Check sheet for the drawn part. Datum: minimum x, y, z corner. Units: mm. Round coordinates to 2 decimals unless told otherwise and drop trailing zeros. Order: outer loops, then holes, each group sorted by start corner. A loop starts at its lowest first (then second) coordinate and runs counter-clockwise, first axis right, second up.
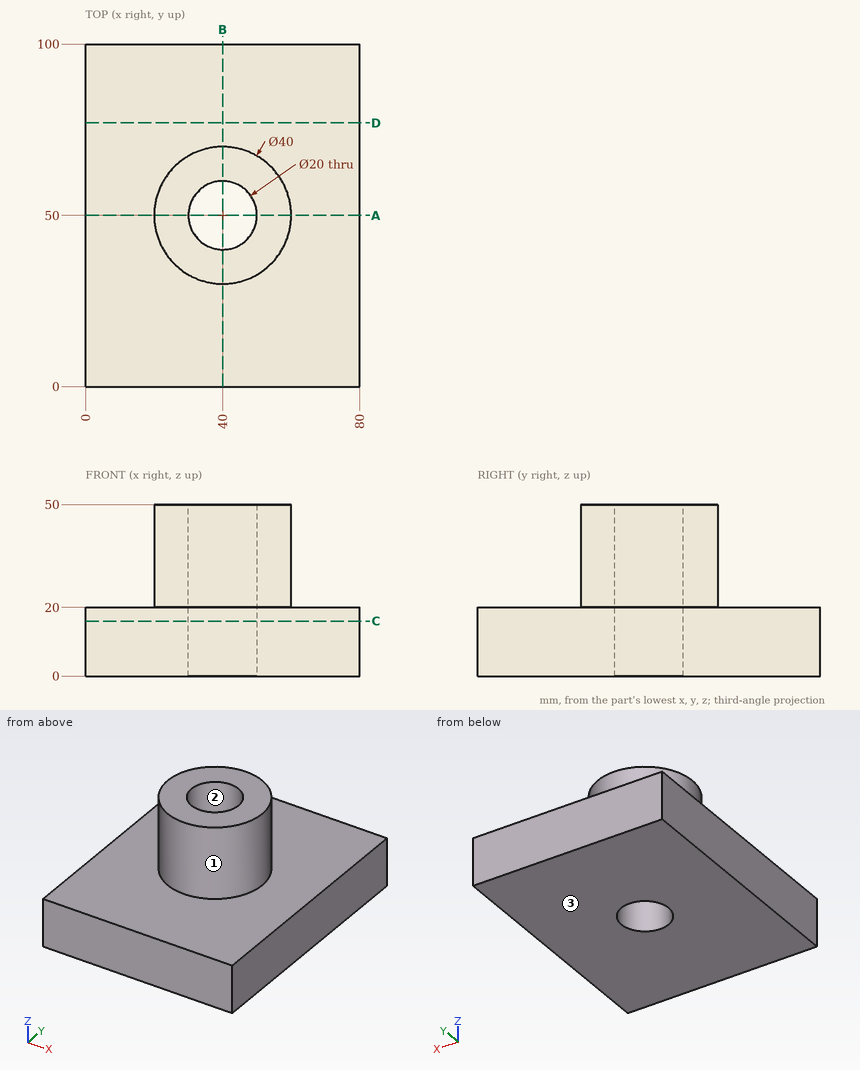
1) Sectioned sample at C-C on z = 16. Record the cut outline in (x, y), and give its area (3 significant figures).
2) Draft check along X on the marked faces 1, 2 and 3. Enter one of: pulls with the +X half, pulls with the -X half, needs draft (parallel to the pull), parting line crosses it, or undercut.
3) Sectioned sample at A-A on y = 50. Record the cut outline in (x, z), and give its area (3 significant figures).
4) Sectioned sample at D-D on y = 77. Record the cut outline in (x, z).
5) Gauge pin test, flat ends, axial feed: pin 1 (6 mm diameter, centred on x = 53.5, z = 24.5, fed in from +Y); pin 2 (10 mm diameter, centred on x = 63, z = 35.5, fed in from +Y); pin 3 (4 mm diameter, centred on y = 44.5, z = 34, fed in from -X). Record the tip position at first contact, or that the pin passes through.
6) Sectioned sample at B-B on x = 40. Record the cut outline in (y, z), and give its area (3 significant figures).
7) Scan lines: line 1 (Y direction, x = 40, z = 10); line 2 (Y direction, x = 40, z = 29); line 3 (Z direction, x = 17, y = 14). Record each from-to range of solid material in increasing order.
Values found:
1. outline: (0, 0) - (80, 0) - (80, 100) - (0, 100) - close; hole circle Ø20 at (40, 50)
1. area: 7,690 mm2
2. face 1: parting line crosses it
2. face 2: undercut
2. face 3: needs draft
3. outline: (0, 0) - (30, 0) - (30, 50) - (20, 50) - (20, 20) - (0, 20) - close; (50, 0) - (80, 0) - (80, 20) - (60, 20) - (60, 50) - (50, 50) - close
3. area: 1,800 mm2
4. outline: (0, 0) - (80, 0) - (80, 20) - (0, 20) - close
5. pin 1: stops at y = 67.02
5. pin 2: stops at y = 58.72
5. pin 3: stops at x = 20.31
6. outline: (0, 0) - (40, 0) - (40, 50) - (30, 50) - (30, 20) - (0, 20) - close; (60, 0) - (100, 0) - (100, 20) - (70, 20) - (70, 50) - (60, 50) - close
6. area: 2,200 mm2
7. line 1: y = 0 to 40, 60 to 100
7. line 2: y = 30 to 40, 60 to 70
7. line 3: z = 0 to 20
